Part model, mm, in its own coordinate system. Face numbers are marked on the shaded views. A direction names the side the tool comes from. Round coordinates to 2 decimals unless told otherwise and drop trailing zeros. Loops run counter-clockwise (first coordinate to the right, second up) from the corner with the lowest first, then second, coordinate; pieces in that order, holes last.
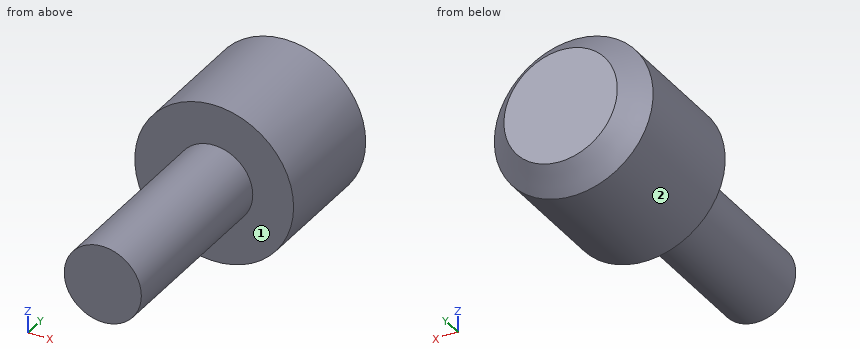
from build123d import *

# Parameters (mm, degrees)
SKETCH1_R           = 3.5
BOSS_EXTRUDE1_DEPTH = 6.5
CHAMFER1_SIZE       = 1
SKETCH2_R           = 1.7
BOSS_EXTRUDE2_DEPTH = 8.5


with BuildPart() as part:
    # Sketch1 → Boss-Extrude1 (new body)
    with BuildSketch(Plane(origin=(0, 0, 0), x_dir=(1, 0, 0), z_dir=(0, 1, 0))):
        Circle(SKETCH1_R)
    extrude(amount=BOSS_EXTRUDE1_DEPTH)

    # Chamfer1
    chamfer1_edges = [part.edges().sort_by_distance(p)[0] for p in [
        (-3.5, 6.5, 0),
    ]]
    chamfer(chamfer1_edges, length=CHAMFER1_SIZE)

    # Sketch2 → Boss-Extrude2 (add)
    with BuildSketch(Plane.XZ):
        Circle(SKETCH2_R)
    extrude(amount=BOSS_EXTRUDE2_DEPTH)


solid = part.part
1) Wall check: line 1 along Y through (x, z) = (2, -1); line 2 along Z through (x, y) = (-1, -2.75); line 3 along X through (y, z) = (2.5, 2.5). Give the ranges that are in metal, low to high.
Values:
line 1: y = 0 to 6.5
line 2: z = -1.37 to 1.37
line 3: x = -2.45 to 2.45
2) Slice it at C-C, the plane y = -3.5. Give the cut face in (x, z), then the cut area to 3 significant figures.
Values:
outline: circle Ø3.4 at (0, 0)
area: 9.08 mm2
3) Drop flat-ended pins along their axis: pin 1 Ø1.5 at (x, z) = (-2, 0) entering from -Y; pin 2 Ø2 at (x, y) = (1.5, 3) entering from -Z. Give the stop position or say it passes through.
Values:
pin 1: stops at y = -8.5
pin 2: stops at z = -3.46
4) Tool access for the marked faces 1 and 2: list every direction of +Z, -Z, +X, -X, +Y, -Y with a clear straight run to the whole face (end or side of a thin tool).
Values:
face 1: -Y
face 2: +Y, -Y
5) Slice it at A-A, the plane z = 0. Give the cut face in (x, y).
Values:
outline: (-3.5, 0) - (-1.7, 0) - (-1.7, -8.5) - (1.7, -8.5) - (1.7, 0) - (3.5, 0) - (3.5, 5.5) - (2.5, 6.5) - (-2.5, 6.5) - (-3.5, 5.5) - close
6) Slice it at B-B, the plane x = 0. Give the cut face in (y, z).
Values:
outline: (-8.5, -1.7) - (0, -1.7) - (0, -3.5) - (5.5, -3.5) - (6.5, -2.5) - (6.5, 2.5) - (5.5, 3.5) - (0, 3.5) - (0, 1.7) - (-8.5, 1.7) - close
7) Slice it at D-D, the plane y = 4.5. Give the cut face in (x, z), then the cut area to 3 significant figures.
Values:
outline: circle Ø7 at (0, 0)
area: 38.5 mm2
